Autodesk Inventor part; units mm, degrees
ref_plane "YZ Plane" through (0, 0, 0) normal (1, 0, 0) x (0, 1, 0)
ref_plane "XZ Plane" through (0, 0, 0) normal (0, 1, 0) x (-1, 0, 0)
ref_plane "XY Plane" through (0, 0, 0) normal (0, 0, 1) x (1, 0, 0)
ref_plane "Arbeitsebene1" through (0, 0, 0) normal (0, 0, 1) x (1, 0, 0)
sketch "Skizze1" plane through (0, 0, 0) normal (0, 0, 1) x (1, 0, 0)
  circle A0 centre (-3.3862, 11.51) radius 1.4
  circle A1 centre (-42.7562, -11.35) radius 1.4
  circle A2 centre (-42.7562, 11.51) radius 1.4
  circle A3 centre (-3.3862, -11.35) radius 1.4
  circle A4 centre (-23.0712, 0.08) radius 13
  line L0 (-6.1126, -24.9) -> (-40.0712, -24.9)
  line L1 (-40.0712, -24.9) -> (-40.0712, -21.3252)
  line L2 (-40.0712, -21.3252) -> (-44.3964, -17)
  line L3 (-44.3964, -17) -> (-47.9712, -17)
  line L4 (-47.9712, -17) -> (-47.9712, 17)
  line L5 (-47.9712, 17) -> (-44.3964, 17)
  line L6 (-44.3964, 17) -> (-40.0712, 21.3252)
  line L7 (-40.0712, 21.3252) -> (-40.0712, 24.9)
  line L8 (-40.0712, 24.9) -> (-6.0712, 24.9)
  line L9 (-6.0712, 24.9) -> (-6.0712, 21.3252)
  line L10 (-6.0712, 21.3252) -> (-1.746, 17)
  line L11 (-1.746, 17) -> (1.8288, 17)
  line L12 (1.8288, 17) -> (1.8288, -17)
  line L13 (1.8288, -17) -> (-1.746, -17)
  line L14 (-1.746, -17) -> (-6.1126, -21.3666)
  line L15 (-6.1126, -21.3666) -> (-6.1126, -24.9)
  point P0 (0, 0)
extrude "Extrusion1" add sketch "Skizze1" along normal blind 1
properties part number "20_Cube_Insert_XY_manipulator_lid_v3"
Work out the finished part from the listing and answer in its coordinate system (mm). Round coordinates to 2 decimals unless told otherwise and drop trailing zeros. Write each loop counter-clockwise with the first axis right and the second up, starting at its lowest first coordinate (ties: lowest second). Pieces come first, ordered by that corner, then holes. Notation, with made-up numbers: (25.25, -5) - (31.25, -5) arc R9 ccw to (31.25, 3) - close; hole circle Ø10 at (-12.5, 86). An arc over 180 degrees is marked (long way). Return JSON: item names as keys, results as strings. Group by question number.
Q1. The mould has two halves that part along X. Classify faces 1 (the cylindrical face through (-36.06, -0.49, 0.49)), 2 (the flat face through (-3.899, -19.153, 0.493)), 3 (the flat face through (-42.204, -19.193, 0.493)): released by +X, released by -X, zero draft, split by the parting line, or undercut.
Q2. The part is cut by section C-C on x = -34. Write down the section's boundary in (y, z), then the cut area to 3 significant figures.
Q3. The part is cut by section A-A on z = 0.75. Write down the section's boundary in (x, y), then the cut area to 3 significant figures.
Q4. Find the intervals of material crossed by L1, parallel to X at y = 12, z = 0.1; L2, parallel to X at y = 4.5, z = 0.75; L3, parallel to Y at x = -30, z = 0.3, in increasing order.
Q5. The part is cut by section D-D on y = -11.35. Write down the section's boundary in (x, z), then the cut area to 3 significant figures.
Q6. Each of these flat-tipped pins is pushed along its axis until it touches: pin 1 Ø3 at (x, y) = (-42.76, 11.51) entering from +Z; pin 2 Ø0.5 at (x, z) = (-0.5, 0.5) entering from +Y; pin 3 Ø0.5 at (x, z) = (-46, 0.5) entering from -Y. Where does it stop, or does it pass through?
Q7. The part is cut by section B-B on y = 0.08. Write down the section's boundary in (x, z).
Solved:
{
 "1": {"face 1": "undercut", "face 2": "released by +X", "face 3": "released by -X"},
 "2": {"outline": "(-24.9, 0) - (-6.96, 0) - (-6.96, 1) - (-24.9, 1) - close; (7.12, 0) - (24.9, 0) - (24.9, 1) - (7.12, 1) - close", "area": "35.7 mm²"},
 "3": {"outline": "(-47.97, -17) - (-44.4, -17) - (-40.07, -21.33) - (-40.07, -24.9) - (-6.11, -24.9) - (-6.11, -21.37) - (-1.75, -17) - (1.83, -17) - (1.83, 17) - (-1.75, 17) - (-6.07, 21.33) - (-6.07, 24.9) - (-40.07, 24.9) - (-40.07, 21.33) - (-44.4, 17) - (-47.97, 17) - close; hole circle Ø2.8 at (-42.76, -11.35); hole circle Ø2.8 at (-42.76, 11.51); hole circle Ø26 at (-23.07, 0.08); hole circle Ø2.8 at (-3.39, -11.35); hole circle Ø2.8 at (-3.39, 11.51)", "area": "1,710 mm²"},
 "4": {"L1": "-47.97 to -44.07, -41.44 to -28.26, -17.88 to -4.7, -2.07 to 1.83", "L2": "-47.97 to -35.3, -10.85 to 1.83", "L3": "-24.9 to -10.92, 11.08 to 24.9"},
 "5": {"outline": "(-47.97, 0) - (-44.16, 0) - (-44.16, 1) - (-47.97, 1) - close; (-41.36, 0) - (-29.26, 0) - (-29.26, 1) - (-41.36, 1) - close; (-16.88, 0) - (-4.79, 0) - (-4.79, 1) - (-16.88, 1) - close; (-1.99, 0) - (1.83, 0) - (1.83, 1) - (-1.99, 1) - close", "area": "31.8 mm²"},
 "6": {"pin 1": "z = 1", "pin 2": "y = 17", "pin 3": "y = -17"},
 "7": {"outline": "(-47.97, 0) - (-36.07, 0) - (-36.07, 1) - (-47.97, 1) - close; (-10.07, 0) - (1.83, 0) - (1.83, 1) - (-10.07, 1) - close"}
}
